Check sheet for the modelled part. Datum: model origin and axes. Units: mm. A direction names the side the tool comes from. Give positions to 0.01 mm unless a question says otherwise; leave off trailing zeros. Order: outer loops, then holes, each group sorted by start corner. A loop starts at its lowest first (then second) coordinate and runs counter-clockwise, first axis right, second up. Notation, with made-up numbers: (12.5, 31.5) - (59.5, 31.5) arc R29 ccw to (59.5, 65.5) - close; hole circle Ø9 at (75, 89.25). An arc over 180 degrees is marked (long way). Answer in a Markdown table with one row per item.
from build123d import *

# Parameters (mm, degrees)
F0_R     = 7.62
F1_DEPTH = 8.89
F0_W     = 85.2932
F0_H     = 54.61
F2_DEPTH = 5.08
F3_R     = 7.62


with BuildPart() as f1:
    # F0 (on Top) → F1 (new body)
    with BuildSketch(Plane.XY):
        Circle(F0_R)
    extrude(amount=F1_DEPTH)

    # F0 (on Top) → F2 (join)
    with BuildSketch(Plane.XY):
        Rectangle(F0_W, F0_H)
        Circle(F0_R, mode=Mode.SUBTRACT)
        Circle(F0_R)
    extrude(amount=-F2_DEPTH)

    # F3
    f3_edges = [f1.edges().sort_by_distance(p)[0] for p in [
        (42.6466, -27.305, -2.54),
        (-42.6466, -27.305, -2.54),
    ]]
    fillet(f3_edges, radius=F3_R)


solid = f1.part
(1) Thickness scan on L1, parallel to Z at x = 13.5, y = -14; L2, parallel to Y at x = -38, z = -4 (3 decimals); L3, parallel to X at y = -2, z = 0.5. Record the ranges inside material, lowest first.
Geometry says:
| item | result |
|---|---|
| L1 | -5.08 to 0 |
| L2 | -26.701 to 27.305 |
| L3 | -7.35 to 7.35 |
(2) Cross-section at D-D, the plane x = -32.5. Record the cut outline in (y, z) (3 decimals), then the cut area to 3 significant figures.
Geometry says:
| item | result |
|---|---|
| outline | (-27.305, -5.08) - (27.305, -5.08) - (27.305, 0) - (-27.305, 0) - close |
| area | 277 mm² |
(3) Cross-section at A-A, the plane y = 0. Record the cut outline in (x, z), then the cut area to 3 significant figures.
Geometry says:
| item | result |
|---|---|
| outline | (-42.65, -5.08) - (42.65, -5.08) - (42.65, 0) - (7.62, 0) - (7.62, 8.89) - (-7.62, 8.89) - (-7.62, 0) - (-42.65, 0) - close |
| area | 569 mm² |
(4) Gauge pin test, flat ends, axial feed: P1, Ø16.5, axis at x = -10.5, y = -7.5, coming from the +Z side; P2, Ø12, axis at x = 17, y = -7, coming from the +Z side. Record the tip position at first contact, or that the pin passes through.
Geometry says:
| item | result |
|---|---|
| P1 | z = 8.89 |
| P2 | z = 0 |
(5) Cross-section at C-C, the plane z = 6.75. Record the cut outline in (x, y).
Geometry says:
| item | result |
|---|---|
| outline | circle Ø15.24 at (0, 0) |
(6) Cross-section at B-B, the plane x = 0. Record the cut outline in (y, z) (3 decimals).
Geometry says:
| item | result |
|---|---|
| outline | (-27.305, -5.08) - (27.305, -5.08) - (27.305, 0) - (7.62, 0) - (7.62, 8.89) - (-7.62, 8.89) - (-7.62, 0) - (-27.305, 0) - close |
(7) Access from +Z, -Z, +X, -X, +Y, -Y to the whole of each face (thin tool, end or side, straight path). Record for faces 1 (the flat face through (-1, 27.305, -3)), 2 (the cylindrical face through (-1.65, -7.44, 4.38)).
Geometry says:
| item | result |
|---|---|
| face 1 | +Z, -Z, +X, -X, +Y |
| face 2 | +Z |
